Could you check a few things on this model? Use its own coordinates, in mm. Face numbers are marked on the shaded views. A direction names the side the tool comes from. Coordinates: 2 decimals unless noted, no trailing zeros. Order: outer loops, then holes, each group sorted by start corner. A loop starts at its lowest first (then second) coordinate and runs counter-clockwise, first axis right, second up. Notation, with made-up numbers: (63.5, -17.75) -> (95.5, -17.75) arc R22 cw to (95.5, -11.75) -> close; hole circle Ø8 at (-6.75, 1). An arc over 180 degrees is marked (long way). Return JSON: item names as keys, results as strings. Group by question number.
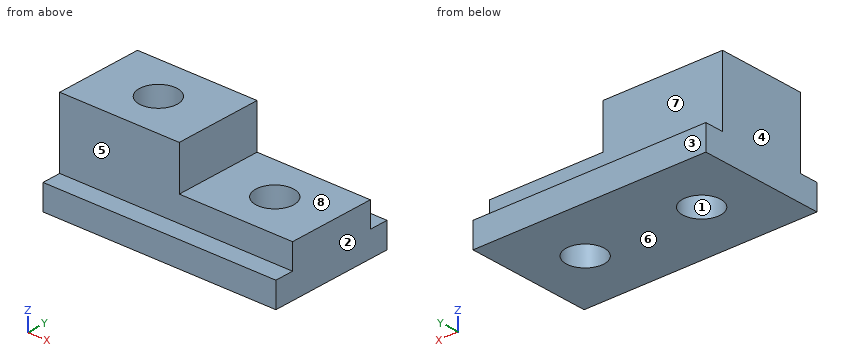
from build123d import *

# Parameters (mm, degrees)
F1_DEPTH = 117.475
F2_R     = 9.525
F3_DEPTH = 161.29
F4_W     = 44.45
F4_H     = 22.225
F5_DEPTH = 57.15


with BuildPart() as f1:
    # F0 (on Right) → F1 (new body)
    with BuildSketch(Plane.YZ):
        Polygon((0, 12.7), (0, 0), (63.5, 0), (63.5, 12.7), (53.975, 12.7), (53.975, 47.625), (9.525, 47.625), (9.525, 12.7), align=None)
    extrude(amount=F1_DEPTH)

    # F2 (on face) → F3 (cut)
    with BuildSketch(Plane.XY.offset(47.625)):
        with Locations((30.1625, 31.75)):
            Circle(F2_R)
        with Locations((88.9, 31.75)):
            Circle(F2_R)
    extrude(amount=-F3_DEPTH, mode=Mode.SUBTRACT)

    # F4 (on face) → F5 (cut)
    with BuildSketch(Plane.YZ.offset(117.475)):
        with Locations((31.75, 36.5125)):
            Rectangle(F4_W, F4_H)
    extrude(amount=-F5_DEPTH, mode=Mode.SUBTRACT)


solid = f1.part
Q1. I want a section at A-A on z = 6.5. State how many separate pieces and enclosed holes the cut face has, and give its area (3 significant figures).
Q2. I'm going to push flat-ended pins straight in: pin 1 Ø5 at (x, z) = (26, 30) entering from +Y (3 decimals); pin 2 Ø1.5 at (x, y) = (54, 50) entering from -Z; pin 3 Ø13.5 at (x, y) = (99.5, 23.5) entering from +Z; pin 4 Ø10 at (x, z) = (45, 34.5) entering from -Y (3 decimals). Where does each tip first touch, or does it pass through?
Q3. On a 3-axis mill with a long thin cutter (end or side, diameter ignored), from which of +Z, -Z, +X, -X, +Y, -Y can I reach the whole of each face in a straight line? I mean the marked faces 5, 6, 7 and 8. Say none if no direction works.
Q4. I need wall thicknesses on line 1 along Y through (x, z) = (88.9, 15.75) (3 decimals); line 2 along Y through (x, z) = (88.9, 9) (3 decimals); line 3 along X through (y, z) = (31, 19) (3 decimals). Which ranges of each line are inside material? Lowest first, please. Write a range as from..to.
Q5. I want a section at B-B on x = 88.9. Please give me the cut outline in (y, z) (3 decimals).
Q6. I want a section at C-C on y = 31.75. Please give me the cut outline in (x, z) (1 decimal).
Q7. We'd pull the mould along X, two halves only. Please class the marked faces 1, 2, 3 and 4: pulls with the +X half, pulls with the -X half, needs draft (parallel to the pull), parting line crosses it, or undercut.
Response values:
{
 "1": {"separate pieces": "1", "enclosed holes": "2", "area": "6,890 mm²"},
 "2": {"pin 1": "stops at y = 53.975", "pin 2": "stops at z = 0", "pin 3": "stops at z = 25.4", "pin 4": "stops at y = 9.525"},
 "3": {"face 5": "+Z, +X, -X, -Y", "face 6": "-Z, +X, -X, +Y, -Y", "face 7": "+Z, +X, -X, +Y", "face 8": "+Z, +X, +Y, -Y"},
 "4": {"line 1": "y = 9.525..22.225, 41.275..53.975", "line 2": "y = 0..22.225, 41.275..63.5", "line 3": "x = 0..20.667, 39.658..79.405, 98.395..117.475"},
 "5": {"outline": "(0, 0) -> (22.225, 0) -> (22.225, 25.4) -> (9.525, 25.4) -> (9.525, 12.7) -> (0, 12.7) -> close; (41.275, 0) -> (63.5, 0) -> (63.5, 12.7) -> (53.975, 12.7) -> (53.975, 25.4) -> (41.275, 25.4) -> close"},
 "6": {"outline": "(0, 0) -> (20.6, 0) -> (20.6, 47.6) -> (0, 47.6) -> close; (39.7, 0) -> (79.4, 0) -> (79.4, 25.4) -> (60.3, 25.4) -> (60.3, 47.6) -> (39.7, 47.6) -> close; (98.4, 0) -> (117.5, 0) -> (117.5, 25.4) -> (98.4, 25.4) -> close"},
 "7": {"face 1": "undercut", "face 2": "pulls with the +X half", "face 3": "needs draft", "face 4": "pulls with the -X half"}
}
